from build123d import *

# Parameters (mm, degrees)
F0_R     = 6.35
F1_DEPTH = 6.35
F2_R     = 0.635
F3_R     = 5.08
F4_DEPTH = 76.2
F5_DEPTH = 76.2
F6_R     = 5.08


with BuildPart() as f1:
    # F0 (on Front) → F1 (new body)
    with BuildSketch(Plane.XZ):
        with BuildLine():
            ThreePointArc((0, 50.8), (-35.921024, -35.921024), (50.8, 0))
            Line((50.8, 0), (0, 0))
            Line((0, 0), (0, 50.8))
        make_face()
        with BuildLine():
            Line((0, 0), (50.8, 0))
            ThreePointArc((50.8, 0), (35.921024, 35.921024), (0, 50.8))
            Line((0, 50.8), (0, 0))
        make_face()
        with Locations((19.05, 25.4)):
            Circle(F0_R, mode=Mode.SUBTRACT)
        with Locations((19.05, 25.4)):
            Circle(F0_R)
    extrude(amount=F1_DEPTH)

    # F2
    f2_edges = [f1.edges().sort_by_distance(p)[0] for p in [
        (-50.8, -6.35, 0),
        (-50.8, 0, 0),
    ]]
    fillet(f2_edges, radius=F2_R)

    # F3 (on face) → F4 (join)
    with BuildSketch(Plane.XZ.offset(6.35)):
        with Locations((20.085614, 24.702994)):
            Circle(F3_R)
    extrude(amount=F4_DEPTH)

    # F3 (on face) → F5 (join)
    with BuildSketch(Plane.XZ.offset(6.35)):
        with Locations((20.085614, 24.702994)):
            Circle(F3_R)
        with Locations((20.771028, -19.2132)):
            Circle(F3_R)
        with Locations((-19.992113, -18.953562)):
            Circle(F3_R)
        with Locations((-18.953562, 26.223423)):
            Circle(F3_R)
    extrude(amount=F5_DEPTH)

    # F6
    f6_edges = [f1.edges().sort_by_distance(p)[0] for p in [
        (-24.033562, -82.55, 26.223423),
        (15.005614, -82.55, 24.702994),
        (-25.072113, -82.55, -18.953562),
        (15.691028, -82.55, -19.2132),
    ]]
    fillet(f6_edges, radius=F6_R)


solid = f1.part
Check sheet for the modelled part. Datum: model origin and axes. Units: mm. Give positions to 0.01 mm unless a question says otherwise; leave off trailing zeros. Write each loop counter-clockwise with the first axis right and the second up, starting at its lowest first coordinate (ties: lowest second). Pieces come first, ordered by that corner, then holes. Notation, with made-up numbers: M 29,67.25 L 77,67.25 A24 ccw 77,89.25 Z; hole C 0.25,20 d1. An arc over 180 degrees is marked long. Use one line per item in the form item = value.
(1) Section check A-A on y = -25. Record the boundary of the cut face in (x, z).
Answer block:
outline = C -19.99,-18.95 d10.16; C -18.95,26.22 d10.16; C 20.09,24.7 d10.16; C 20.77,-19.21 d10.16
(2) Material ranges on line 1 along Z through (x, y) = (20.5, -68); line 2 along Y through (x, z) = (35, 32); line 3 along Z through (x, y) = (23, -15), recorded low to high.
Answer block:
line_1 = -24.29 to -14.14, 19.64 to 29.77
line_2 = -6.35 to 0
line_3 = -23.78 to -14.65, 20.54 to 28.86
(3) Depth check by flat-ended pin: P1, Ø10, axis at x = 16, z = -27.5, coming from the -Y side; P2, Ø4, axis at x = 21, z = 4.5, coming from the -Y side; P3, Ø10, axis at y = -38.5, z = -16, coming from the -X side. Enter the tip coordinate at first touch or a pass-through.
Answer block:
P1 = -79.7
P2 = -6.35
P3 = -25.07
(4) Draft check along Z on faces 1 (the flat face through (-1, 0, 1)), 2 (the cylindrical face through (24.93, -41.41, 26.23)). Enter one of: pulls with the +Z half, pulls with the -Z half, needs draft (parallel to the pull), parting line crosses it, or undercut.
Answer block:
face_1 = needs draft
face_2 = undercut
